Build history of the part. All positions in model axes, mm. Face numbers are marked on the shaded views. A direction names the side the tool comes from. Give positions to 0.01 mm unless a question says otherwise; leave off trailing zeros. Order: outer loops, then holes, each group sorted by start corner. A loop starts at its lowest first (then second) coordinate and runs counter-clockwise, first axis right, second up. Notation, with made-up numbers: M 82.25,24 L 99.25,24 A26 ccw 99.25,48 Z; hole C 63,69 d2. An arc over 180 degrees is marked long. Use CSV: the item, a comma, the result in double quotes. Start each with the question number.
Item 1: Band-saw the part on D-D on x = -20. Write the cut outline in (y, z), plus the area to 3 significant figures.
Item 2: Band-saw the part on C-C on z = 10.75. Write the cut outline in (x, y).
Item 3: Pin check, flat tips, straight feed: P1, Ø1, axis at x = -8, z = 2.5, coming from the +Y side; P2, Ø6, axis at x = -16, y = 12.5, coming from the -Z side; P3, Ø25, axis at x = 6, y = 7, coming from the -Z side; P4, Ø5, axis at x = 3.5, z = 11.5, coming from the -Y side. Stop position of each tip, or through.
Item 4: Wall check: line 1 along Y through (x, z) = (0, 10); line 2 along Y through (x, z) = (0, 6.5); line 3 along Z through (x, y) = (-4.5, 17.5). Give the ranges that are in metal, low to high.
Item 5: Which spindle directions (+Z, -Z, +X, -X, +Y, -Y) get a long thin tool onto all of the face, cutting with end or side? Do the marked faces 1 and 2. Say none if no direction does.
Item 6: Band-saw the part on A-A on y = 0. Write the cut outline in (x, z), plus the area to 3 significant figures.
from build123d import *

# Parameters (mm, degrees)
ESQUISSE1_R             = 11.5
BOSS_EXTRU_1_DEPTH      = 13
ESQUISSE2_R             = 25
ESQUISSE2_R_2           = 7.5
BOSS_EXTRU_2_DEPTH      = 6
ESQUISSE5_R             = 7.6
ENL_V_MAT_EXTRU_1_DEPTH = 38.669616404


with BuildPart() as part:
    # Esquisse1 → Boss.-Extru.1 (new body)
    with BuildSketch(Plane.XY):
        with Locations(Location((0, 0, 0), (0, 0, 180))):
            Circle(ESQUISSE1_R)
    extrude(amount=BOSS_EXTRU_1_DEPTH)

    # Esquisse2 → Boss.-Extru.2 (add)
    with BuildSketch(Plane.XY.offset(13)):
        Circle(ESQUISSE2_R)
        Circle(ESQUISSE2_R_2, mode=Mode.SUBTRACT)
    extrude(amount=-BOSS_EXTRU_2_DEPTH)

    # Esquisse5 → Enlèv. mat.-Extru.1 (cut, through all)
    with BuildSketch(Plane.XY.offset(13)):
        Circle(ESQUISSE5_R)
    extrude(amount=-ENL_V_MAT_EXTRU_1_DEPTH, mode=Mode.SUBTRACT)


solid = part.part
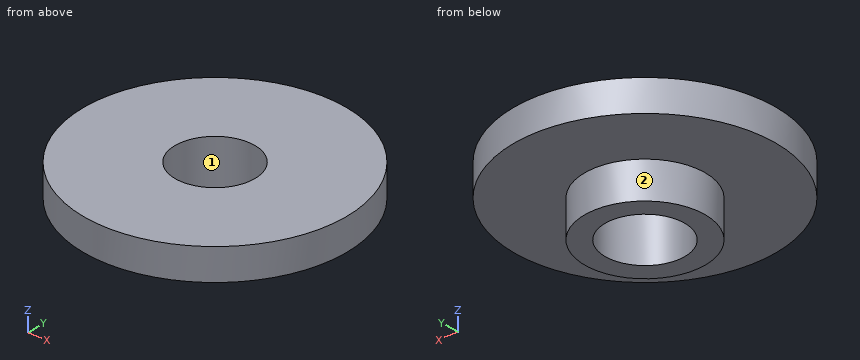
Model answer:
1,outline,"M -15,7 L 15,7 L 15,13 L -15,13 Z"
1,area,"180 mm^2"
2,outline,"C 0,0 d50; hole C 0,0 d15.2"
3,P1,"stops at y = 8.72"
3,P2,"stops at z = 7"
3,P3,"stops at z = 0"
3,P4,"stops at y = -24.98"
4,line 1,"y = -25 to -7.6, 7.6 to 25"
4,line 2,"y = -11.5 to -7.6, 7.6 to 11.5"
4,line 3,"z = 7 to 13"
5,face 1,"+Z, -Z"
5,face 2,"-Z"
6,outline,"M -25,7 L -11.5,7 L -11.5,0 L -7.6,0 L -7.6,13 L -25,13 Z; M 7.6,0 L 11.5,0 L 11.5,7 L 25,7 L 25,13 L 7.6,13 Z"
6,area,"263 mm^2"
